```python
from build123d import *

# Parameters (mm, degrees)
SKETCH2_W           = 120
SKETCH2_H           = 100
BOSS_EXTRUDE1_DEPTH = 2.5
SKETCH3_W           = 114.9
SKETCH3_H           = 94.9
SKETCH3_W_2         = 111.9
SKETCH3_H_2         = 91.9
BOSS_EXTRUDE2_DEPTH = 5
SKETCH4_W           = 71.17
SKETCH4_H           = 71.17
SKETCH4_W_2         = 40
SKETCH4_H_2         = 14
CUT_EXTRUDE1_DEPTH  = 2.5


with BuildPart() as part:
    # Sketch2 → Boss-Extrude1 (new body)
    with BuildSketch(Plane.XY):
        Rectangle(SKETCH2_W, SKETCH2_H)
    extrude(amount=BOSS_EXTRUDE1_DEPTH)

    # Sketch3 → Boss-Extrude2 (add)
    with BuildSketch(Plane(origin=(0, 0, 0), x_dir=(-1, 0, 0), z_dir=(0, 0, -1))):
        Rectangle(SKETCH3_W, SKETCH3_H)
        Rectangle(SKETCH3_W_2, SKETCH3_H_2, mode=Mode.SUBTRACT)
    extrude(amount=BOSS_EXTRUDE2_DEPTH)

    # Sketch4 → Cut-Extrude1 (cut)
    with BuildSketch(Plane(origin=(0, 0, 0), x_dir=(-1, 0, 0), z_dir=(0, 0, -1))):
        with Locations((-20.365, 10.365)):
            Rectangle(SKETCH4_W, SKETCH4_H)
        with Locations((-34.95, -37.95)):
            Rectangle(SKETCH4_W_2, SKETCH4_H_2)
    extrude(amount=-CUT_EXTRUDE1_DEPTH, mode=Mode.SUBTRACT)


solid = part.part
```
Input: part model. Units: mm. Frame: model coordinates. A direction names the side the tool comes from. Round coordinates to 2 decimals unless told otherwise and drop trailing zeros. Order: outer loops, then holes, each group sorted by start corner. A loop starts at its lowest first (then second) coordinate and runs counter-clockwise, first axis right, second up. Notation, with made-up numbers: (16.5, 29) - (51.5, 29) arc R27 cw to (51.5, 54) - close; hole circle Ø11 at (44, 0.25). An arc over 180 degrees is marked (long way). Answer in a Markdown table with one row per item.
Item 1: Section query B-B (z = -2.5). Return the cut outline in (x, y).
Model answer:
| item | result |
|---|---|
| outline | (-57.45, -47.45) - (57.45, -47.45) - (57.45, 47.45) - (-57.45, 47.45) - close; hole (-55.95, -45.95) - (55.95, -45.95) - (55.95, 45.95) - (-55.95, 45.95) - close |
Item 2: Section query D-D (x = -10). Return the cut outline in (y, z).
Model answer:
| item | result |
|---|---|
| outline | (-50, 0) - (-47.45, 0) - (-47.45, -5) - (-45.95, -5) - (-45.95, 0) - (-25.22, 0) - (-25.22, 2.5) - (-50, 2.5) - close; (45.95, -5) - (47.45, -5) - (47.45, 0) - (50, 0) - (50, 2.5) - (45.95, 2.5) - close |
Item 3: Mould query, pull axis X, two halves, no side actions, for faces 6 (the flat face through (-28, -10, 2.5)), 7 (the flat face through (35, -30.95, 1)), 8 (the flat face through (-60, -1, 1)). Classes: released by +X, released by -X, zero draft, split by the parting line, or undercut.
Model answer:
| item | result |
|---|---|
| face 6 | zero draft |
| face 7 | undercut |
| face 8 | released by -X |
Item 4: Line query: line 1 (Y direction, x = 48, z = 0.5); line 2 (X direction, y = -3, z = -3.5); line 3 (Y direction, x = -40, z = -1). Output: solid intervals per line, ascending.
Model answer:
| item | result |
|---|---|
| line 1 | y = -50 to -44.95, -30.95 to -25.22, 45.95 to 50 |
| line 2 | x = -57.45 to -55.95, 55.95 to 57.45 |
| line 3 | y = -47.45 to -45.95, 45.95 to 47.45 |
Item 5: Section query C-C (x = 41). Return the cut outline in (y, z).
Model answer:
| item | result |
|---|---|
| outline | (-50, 0) - (-47.45, 0) - (-47.45, -5) - (-45.95, -5) - (-45.95, 0) - (-44.95, 0) - (-44.95, 2.5) - (-50, 2.5) - close; (-30.95, 0) - (-25.22, 0) - (-25.22, 2.5) - (-30.95, 2.5) - close; (45.95, -5) - (47.45, -5) - (47.45, 0) - (50, 0) - (50, 2.5) - (45.95, 2.5) - close |
Item 6: Reachability of faces 1 (the flat face through (-57.45, -1, -2)), 2 (the flat face through (1, 47.45, -2)), 3 (the flat face through (-55.95, -1, -2)), 4 (the flat face through (57.45, -1, -2)), 5 (the flat face through (35, -44.95, 1)) from +Z, -Z, +X, -X, +Y, -Y: full face, straight path, thin tool, end or side. Return the list, or none.
Model answer:
| item | result |
|---|---|
| face 1 | -Z, -X, +Y, -Y |
| face 2 | -Z, +X, -X, +Y |
| face 3 | -Z |
| face 4 | -Z, +X, +Y, -Y |
| face 5 | +Z, -Z |
Item 7: Section query A-A (y = 42). Return the cut outline in (x, z).
Model answer:
| item | result |
|---|---|
| outline | (-60, 0) - (-57.45, 0) - (-57.45, -5) - (-55.95, -5) - (-55.95, 0) - (-15.22, 0) - (-15.22, 2.5) - (-60, 2.5) - close; (55.95, -5) - (57.45, -5) - (57.45, 0) - (60, 0) - (60, 2.5) - (55.95, 2.5) - close |
Item 8: Pin query (flat end, axial travel): pin 1 (2.5 mm diameter, centred on x = -12.5, z = -2.5, fed in from +Y); pin 2 (2.5 mm diameter, centred on y = -10, z = -2.5, fed in from +X); pin 3 (6 mm diameter, centred on x = -46.5, y = 0, fed in from -Z). Return the tip coordinate at first contact, or that it passes through.
Model answer:
| item | result |
|---|---|
| pin 1 | stops at y = 47.45 |
| pin 2 | stops at x = 57.45 |
| pin 3 | stops at z = 0 |
